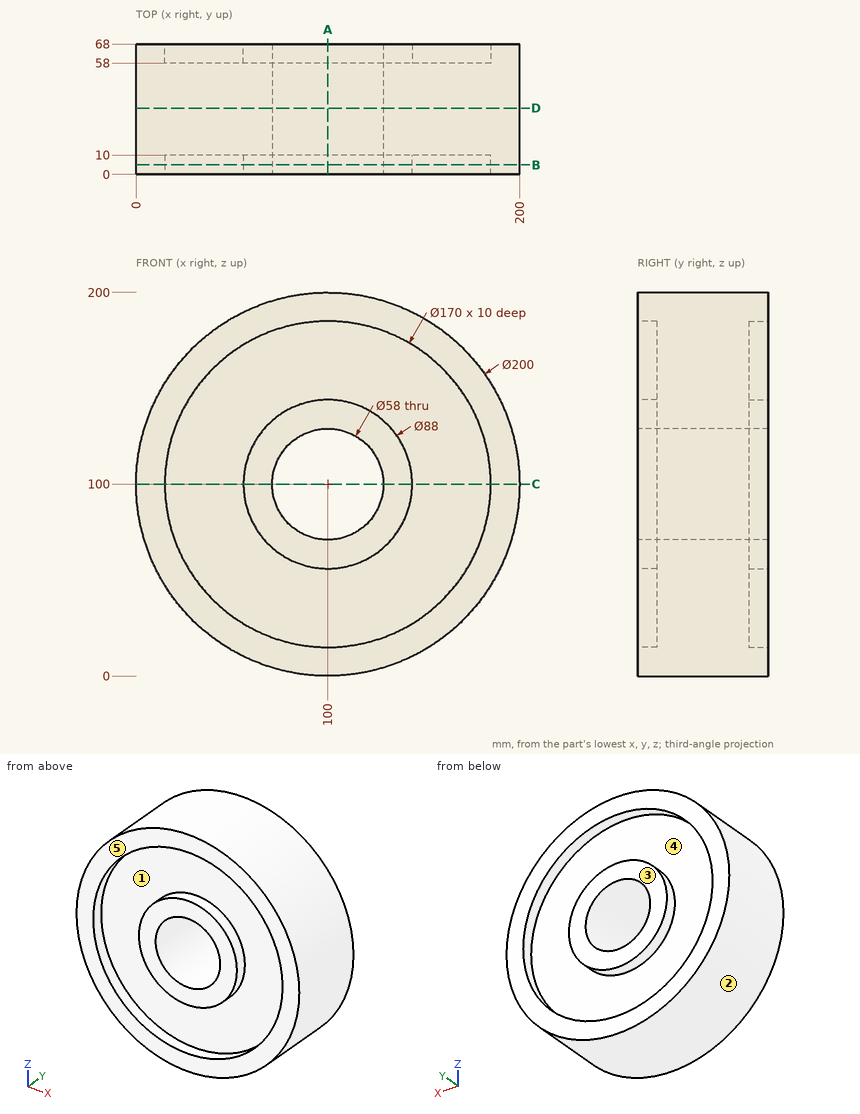
Study the drawing (mm; zero at the part's minimum x, y, z) and answer. A direction names the side the tool comes from. Round coordinates to 2 decimals unless told otherwise and drop trailing zeros. Write each loop counter-clockwise with the first axis right and the second up, starting at its lowest first coordinate (ties: lowest second). Pieces come first, ordered by that corner, then holes. Notation, with made-up numbers: (-1, 4.5) -> (11, 4.5) arc R6 cw to (11, 9.5) -> close; hole circle Ø1 at (23, 65.5). An arc over 180 degrees is marked (long way). Use CSV: the item, a comma, the result in double quotes. Start each with the question number.
(1) Section A-A on x = 100 is taken. Give the vertices of the cut face in (y, z).
(2) Each of these flat-tipped pins is pushed along its axis until it touches: pin 1 (5 mm diameter, centred on y = 43.5, z = 140.5, fed in from -X); pin 2 (3 mm diameter, centred on y = 8.5, z = 135.5, fed in from -X); pin 3 (1 mm diameter, centred on x = 52.5, y = 41, fed in from +Z). Where does it stop, or does it pass through?
(3) Section D-D on y = 34.5 is taken. Give the vertices of the cut face in (x, z).
(4) The mould has two halves that part along Z. Classify the marked faces 1, 2 and 3: released by +Z, released by -Z, zero draft, split by the parting line, or undercut.
(5) Consider L1, parallel to Z at x = 100, y = 63; L2, parallel to X at y = 48, z = 100. Determine where each line is inside the solid, lowest interval first. Write a range as from..to.
(6) Section C-C on z = 100 is taken. Give the vertices of the cut face in (x, y).
(7) Which of the six approach directions +Z, -Z, +X, -X, +Y, -Y give full straight-line access (tool end or side, diameter ignored) to the marked faces 4 and 5?
(8) Section B-B on y = 5 is taken. Give the vertices of the cut face in (x, z).
A:
1,outline,"(0, 0) -> (68, 0) -> (68, 15) -> (58, 15) -> (58, 56) -> (68, 56) -> (68, 71) -> (0, 71) -> (0, 56) -> (10, 56) -> (10, 15) -> (0, 15) -> close; (0, 129) -> (68, 129) -> (68, 144) -> (58, 144) -> (58, 185) -> (68, 185) -> (68, 200) -> (0, 200) -> (0, 185) -> (10, 185) -> (10, 144) -> (0, 144) -> close"
2,pin 1,"stops at x = 7.5"
2,pin 2,"stops at x = 5.96"
2,pin 3,"stops at z = 188.27"
3,outline,"circle Ø200 at (100, 100); hole circle Ø58 at (100, 100)"
4,face 1,"undercut"
4,face 2,"split by the parting line"
4,face 3,"zero draft"
5,L1,"z = 0..15, 56..71, 129..144, 185..200"
5,L2,"x = 0..71, 129..200"
6,outline,"(0, 0) -> (15, 0) -> (15, 10) -> (56, 10) -> (56, 0) -> (71, 0) -> (71, 68) -> (56, 68) -> (56, 58) -> (15, 58) -> (15, 68) -> (0, 68) -> close; (129, 0) -> (144, 0) -> (144, 10) -> (185, 10) -> (185, 0) -> (200, 0) -> (200, 68) -> (185, 68) -> (185, 58) -> (144, 58) -> (144, 68) -> (129, 68) -> close"
7,face 4,"+Y"
7,face 5,"+Z, -Z, +X, -X, -Y"
8,outline,"circle Ø200 at (100, 100); circle Ø88 at (100, 100); hole circle Ø170 at (100, 100); hole circle Ø58 at (100, 100)"
